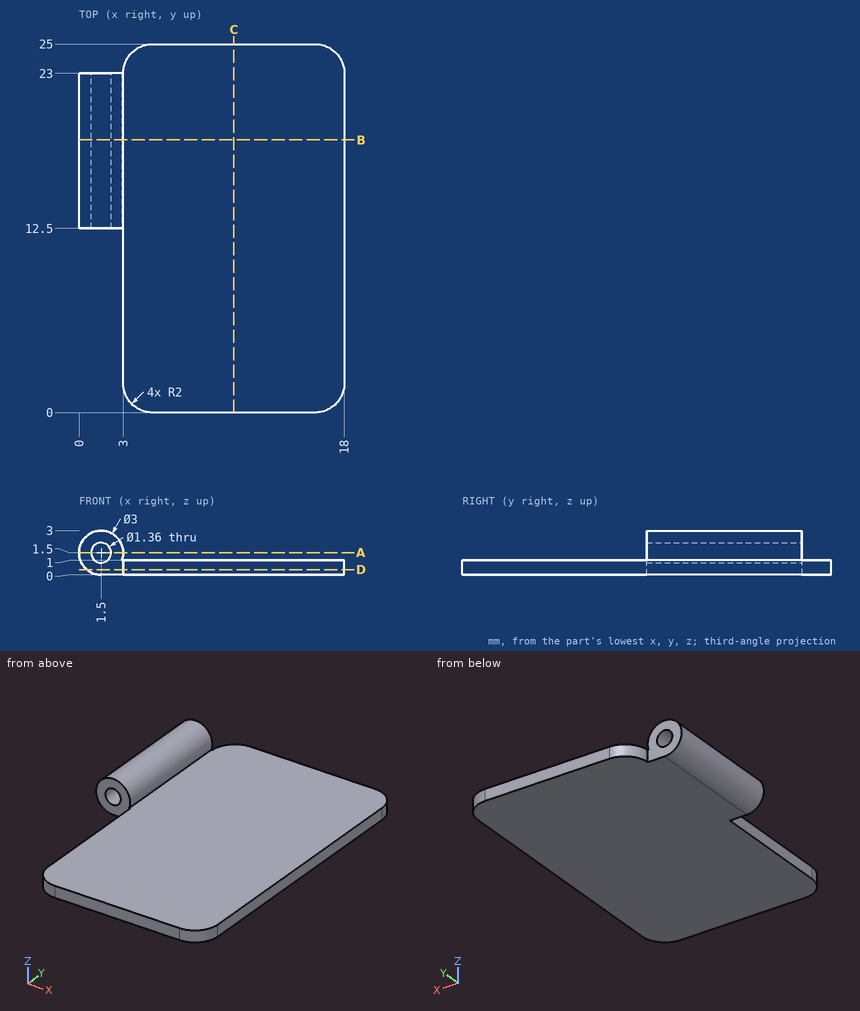
Part print with two shaded views. Sizes in mm from the minimum x, y, z corner. Coordinates: 2 decimals unless noted, no trailing zeros. Order: outer loops, then holes, each group sorted by start corner. A loop starts at its lowest first (then second) coordinate and runs counter-clockwise, first axis right, second up. Notation, with made-up numbers: M 4.25,-18.5 L 36.25,-18.5 A21 cw 36.25,6.5 Z; hole C -27.5,20.5 d3. An arc over 180 degrees is marked long. Use a Markdown table: item, result.
(1) Probe L1, parallel to X at y = 15.75, z = 1.5; L2, parallel to X at y = 3.25, z = 0.3. List the from-to ranges inside material, lowest first.
A:
| item | result |
|---|---|
| L1 | x = 0 to 0.82, 2.18 to 3 |
| L2 | x = 3 to 18 |
(2) Cut at B-B on y = 18.5. Write the cut outline in (x, z).
A:
| item | result |
|---|---|
| outline | M 1.5,0 L 18,0 L 18,1 L 2.91,1 A1.5 ccw long Z; hole C 1.5,1.5 d1.36 |
(3) Cut at C-C on x = 10.5. Write the cut outline in (y, z).
A:
| item | result |
|---|---|
| outline | M 0,0 L 25,0 L 25,1 L 0,1 Z |
(4) Cut at D-D on z = 0.35. Write the cut outline in (x, y).
A:
| item | result |
|---|---|
| outline | M 0.54,12.5 L 3,12.5 L 3,2 A2 ccw 5,0 L 16,0 A2 ccw 18,2 L 18,23 A2 ccw 16,25 L 5,25 A2 ccw 3,23 L 0.54,23 Z |
(5) Flat gauge pins, fed straight in: pin 1 (1.5 mm diameter, centred on x = 4.5, y = 5.5, fed in from +Z); pin 2 (1.5 mm diameter, centred on y = 10, z = 2.5, fed in from -X); pin 3 (1.6 mm diameter, centred on x = 1.5, z = 1.5, fed in from -Y); pin 4 (1.5 mm diameter, centred on x = 1.5, z = 1, fed in from +Y). Where does each tip first touch, or does it go through?
A:
| item | result |
|---|---|
| pin 1 | stops at z = 1 |
| pin 2 | passes through |
| pin 3 | stops at y = 12.5 |
| pin 4 | stops at y = 23 |
(6) Cut at A-A on z = 1.5. Write the cut outline in (x, y), then the cut area to 3 significant figures.
A:
| item | result |
|---|---|
| outline | M 0,12.5 L 0.82,12.5 L 0.82,23 L 0,23 Z; M 2.18,12.5 L 3,12.5 L 3,23 L 2.18,23 Z |
| area | 17.2 mm^2 |
